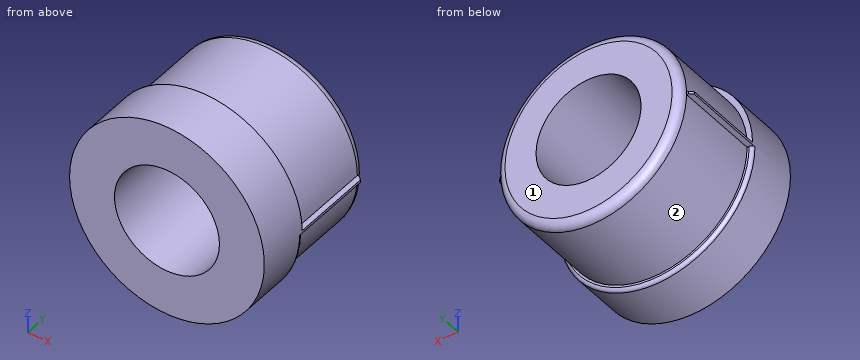
Autodesk Inventor part; units mm, degrees
ref_plane "YZ Plane" through (0, 0, 0) normal (1, 0, 0) x (0, 1, 0)
ref_plane "XZ Plane" through (0, 0, 0) normal (0, 1, 0) x (-1, 0, 0)
ref_plane "XY Plane" through (0, 0, 0) normal (0, 0, 1) x (1, 0, 0)
sketch "Sketch1" plane through (0, 0, 0) normal (0, 1, 0) x (-1, 0, 0)
  circle A0 centre (0, 0) radius 14.732
  dimension "d0" = 29.464
extrude "Extrusion1" add sketch "Sketch1" along normal blind 7.9248
sketch "Sketch2" plane through (0, 7.9248, 0) normal (0, 1, 0) x (1, 0, 0)
  circle A0 centre (0, 0) radius 14.732
  circle A1 centre (0, 0) radius 13.9065
  dimension "d3" = 27.813
extrude "Extrusion2" add sketch "Sketch2" along normal blind 13.97 contours A1
sketch "Sketch4" plane through (0, 7.9248, 0) normal (0, 1, 0) x (1, 0, 0)
  circle A0 centre (0, 0) radius 13.9065
  circle A1 centre (0, 0) radius 14.732
  circle A2 centre (0, 0) radius 13.9065
  circle A3 centre (0, 0) radius 14.732
  line L0 (-13.905, 0.2046) -> (-13.0794, 0.2046) construction
  line L1 (-13.9052, 0.1905) -> (-14.7308, 0.1905)
  line L2 (-13.9052, 0.1905) -> (-13.0796, 0.1905) construction
  line L3 (-13.9052, -0.1905) -> (-14.7308, -0.1905)
  line L4 (-13.9052, -0.1905) -> (-13.0796, -0.1905) construction
  line L5 (-13.9052, 0.1905) -> (14.7308, 0.1896)
  line L6 (-13.9052, -0.1905) -> (14.7307, -0.1927)
  dimension "d7" = 180
  dimension "d8" = 180
extrude "Extrusion3" add sketch "Sketch4" along normal blind 12.7 contours L5 A0 L6 | A0 L3 A1 L1 | L5 A1 L6 A0
chamfer "Chamfer1" distance 0.508 angle 45 1 edges at (14.732, 20.6248, 0.0015)
chamfer "Chamfer2" distance 0.508 angle 45 1 edges at (-14.732, 20.6248, 0)
fillet "Fillet1" radius 1.27 1 edges at (-13.9065, 21.8948, 0)
fillet "Fillet2" radius 0.508 1 edges at (0.0004, 7.9248, -14.732)
sketch "Sketch5" plane through (0, 21.8948, 0) normal (0, 1, 0) x (1, 0, 0)
  circle A0 centre (0, 0) radius 12.6365
  circle A1 centre (0, 0) radius 7.9375
  dimension "d19" = 15.875
extrude "Extrusion4" cut sketch "Sketch5" against normal blind 25.4 contours A1
properties part number "Pipe T with a hole in it"
The model under review builds one solid part; all positions refer to its coordinate system, in mm. Face numbers are marked on the shaded views. A direction names the side the tool comes from. Round coordinates to 2 decimals unless told otherwise and drop trailing zeros. Loops run counter-clockwise (first coordinate to the right, second up) from the corner with the lowest first, then second, coordinate; pieces in that order, holes last.
1) Wall thickness on line 1 along Z through (x, y) = (0, 11); line 2 along Z through (x, y) = (0, 6.75): over which ranges is each line inside the solid? List them lowest first.
Values follow:
line 1: z = -13.91 to -7.94, 7.94 to 13.91
line 2: z = -14.73 to -7.94, 7.94 to 14.73
2) Tool access review of the marked faces 1 and 2: name each direction out of +Z, -Z, +X, -X, +Y, -Y from which nothing blocks a thin tool from reaching the whole face with its end or side.
Values follow:
face 1: +Z, -Z, +X, -X, +Y
face 2: +Y
3) Clearance check with flat-ended pins moving along their axes: P1, Ø7, axis at x = -5.5, z = -5, coming from the +Y side; P2, Ø0.7, axis at x = -14.5, y = 17.5, coming from the +Z side; P3, Ø2, axis at x = 9, z = 11, coming from the +Y side; P4, Ø5, axis at x = -2.5, y = 12.5, coming from the +Z side. State where each tip first meets the part, or that it passes through.
Values follow:
P1: stops at y = 21.89
P2: stops at z = 0.19
P3: stops at y = 21.76
P4: stops at z = 13.91
4) Consider section B-B on x = 0. State the section outline as (y, z) points, then the cut area to 3 significant figures.
Values follow:
outline: (0, -14.73) - (7.42, -14.73) arc R0.51 ccw to (7.92, -14.22) - (7.92, -13.91) - (20.62, -13.91) arc R1.27 ccw to (21.89, -12.64) - (21.89, -7.94) - (0, -7.94) - close; (0, 7.94) - (21.89, 7.94) - (21.89, 12.64) arc R1.27 ccw to (20.62, 13.91) - (7.92, 13.91) - (7.92, 14.73) - (0, 14.73) - close
area: 274 mm2
5) Consider section C-C on y = 5.25. State the section outline as (x, z) points (1 decimal).
Values follow:
outline: circle Ø29.5 at (0, 0); hole circle Ø15.9 at (0, 0)
